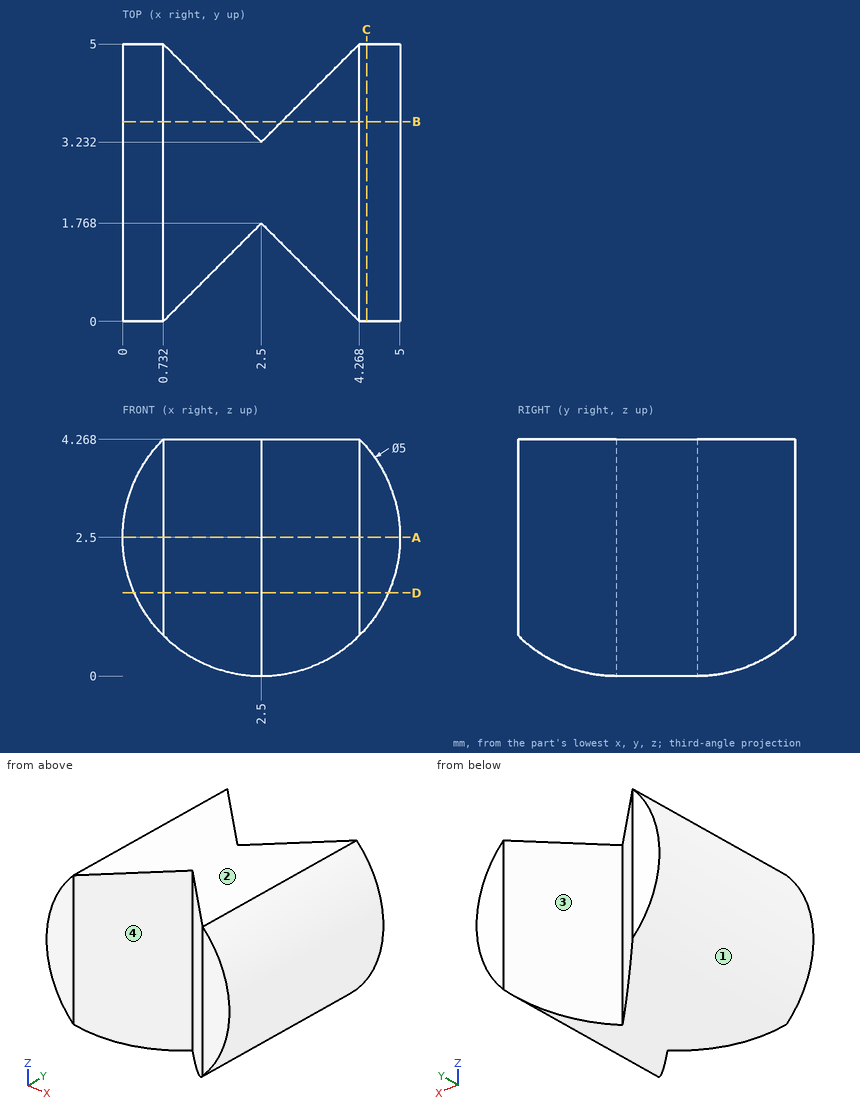
Geometry check sheet. Reference: drawing and pictorial views, mm from the part's lowest x, y, z. Round coordinates to 2 decimals unless told otherwise and drop trailing zeros. Loops run counter-clockwise (first coordinate to the right, second up) from the corner with the lowest first, then second, coordinate; pieces in that order, holes last. Notation, with made-up numbers: (39.25, 85.5) -> (73.25, 85.5) arc R9 ccw to (73.25, 98.5) -> close; hole circle Ø8 at (-1, -8.75). An arc over 180 degrees is marked (long way). Answer as a JSON object with one key per item and string values. Group by question number.
Item 1: Cross-section at A-A, the plane z = 2.5. Record the cut outline in (x, y).
Item 2: Release check for a two-part mould opening along X. For the marked faces 1, 2, 3 and 4 record: pulls with the +X half, pulls with the -X half, needs draft (parallel to the pull), parting line crosses it, or undercut.
Item 3: Cross-section at B-B, the plane y = 3.6. Record the cut outline in (x, z).
Item 4: Depth check by flat-ended pin: pin 1 Ø2 at (x, z) = (2, 2.5) entering from +Y. Enter the tip coordinate at first touch or a pass-through.
Item 5: Cross-section at C-C, the plane x = 4.4. Record the cut outline in (y, z) (1 decimal).
Item 6: Thickness scan on line 1 along X through (y, z) = (4.2, 2.65) (1 decimal); line 2 along X through (y, z) = (4.15, 1.35); line 3 along Y through (x, z) = (3.05, 0.9). Record the ranges inside material, lowest first.
Item 7: Cross-section at D-D, the plane z = 1.5. Record the cut outline in (x, y), plus the area to 3 significant figures.
Determined:
{
 "1": {"outline": "(0, 0) -> (0.73, 0) -> (2.5, 1.77) -> (4.27, 0) -> (5, 0) -> (5, 5) -> (4.27, 5) -> (2.5, 3.23) -> (0.73, 5) -> (0, 5) -> close"},
 "2": {"face 1": "parting line crosses it", "face 2": "needs draft", "face 3": "undercut", "face 4": "undercut"},
 "3": {"outline": "(0.73, 4.27) arc R2.5 ccw to (2.13, 0.03) -> (2.13, 4.27) -> close; (2.87, 0.03) arc R2.5 ccw to (4.27, 4.27) -> (2.87, 4.27) -> close"},
 "4": {"pin 1": "stops at y = 4.73"},
 "5": {"outline": "(0, 0.9) -> (5, 0.9) -> (5, 4.1) -> (0, 4.1) -> close"},
 "6": {"line 1": "x = 0 to 1.5, 3.5 to 5", "line 2": "x = 0.28 to 1.58, 3.42 to 4.72", "line 3": "y = 1.22 to 3.78"},
 "7": {"outline": "(0.21, 0) -> (0.73, 0) -> (2.5, 1.77) -> (4.27, 0) -> (4.79, 0) -> (4.79, 5) -> (4.27, 5) -> (2.5, 3.23) -> (0.73, 5) -> (0.21, 5) -> close", "area": "16.7 mm²"}
}
